Autodesk Inventor part; units mm, degrees
ref_plane "YZ Plane" through (0, 0, 0) normal (1, 0, 0) x (0, 1, 0)
ref_plane "XZ Plane" through (0, 0, 0) normal (0, 1, 0) x (-1, 0, 0)
ref_plane "XY Plane" through (0, 0, 0) normal (0, 0, 1) x (1, 0, 0)
sketch "Sketch1" plane through (0, 0, 0) normal (1, 0, 0) x (0, 1, 0)
  line L0 (0, 0) -> (200, 0)
  line L1 (200, 0) -> (200, -200)
  line L2 (200, -200) -> (0, -200)
  line L3 (0, -200) -> (0, 0)
  dimension "d0" = 200
  dimension "d1" = 200
extrude "Extrusion1" add sketch "Sketch1" along normal blind 6
sketch "Sketch2" plane through (6, 0, 0) normal (1, 0, 0) x (0, 0, -1)
  line L0 (0, 200) -> (0, 0)
  line L1 (0, 0) -> (200, 0)
  line L2 (200, 0) -> (200, 200)
  line L3 (200, 200) -> (0, 200)
  circle A0 centre (50, 130) radius 10
  circle A1 centre (150, 130) radius 10
  circle A2 centre (100, 50) radius 10
  dimension "d4" = 20
  dimension "d5" = 20
  dimension "d6" = 20
  dimension "d7" = 100
  dimension "d8" = 50
  dimension "d9" = 80
  dimension "d10" = 100
  dimension "d11" = 50
  dimension "d12" = 80
extrude "Extrusion2" add sketch "Sketch2" along normal blind 11.1 contours A0 | A1 | A2
sketch "Sketch3" plane through (0, 0, 0) normal (-1, 0, 0) x (0, 0, 1)
  line L0 (0, 0) -> (0, 200)
  line L1 (0, 200) -> (-200, 200)
  line L2 (-200, 200) -> (-200, 0)
  line L3 (-200, 0) -> (0, 0)
  line L4 (-110, 110) -> (-90, 110)
  line L5 (-90, 110) -> (-90, 90)
  line L6 (-90, 90) -> (-110, 90)
  line L7 (-110, 90) -> (-110, 110)
  dimension "d15" = 20
  dimension "d16" = 20
  dimension "d17" = 90
  dimension "d18" = 90
extrude "Extrusion3" add sketch "Sketch3" along normal blind 20 contours L4 L5 L6 L7
sketch "Sketch4" plane through (0, 110, -90) normal (0, 1, 0) x (1, 0, 0)
  line L0 (0, 20) -> (0, 0)
  line L1 (0, 20) -> (-20, 20)
  line L2 (-20, 0) -> (-20, 20)
  line L3 (0, 0) -> (-20, 0)
  line L4 (-20, 0) -> (0, 0)
  line L5 (0, 0) -> (0, 20)
  line L6 (0, 20) -> (-20, 20)
  line L7 (-20, 20) -> (-20, 0)
  point P0 (0, -90)
extrude "Extrusion4" add sketch "Sketch4" along normal blind 200
sketch "Sketch5" plane through (-20, 90, -90) normal (0, 0, 1) x (1, 0, 0)
  line L0 (20, 110) -> (20, 0)
  line L1 (20, 110) -> (20, 220)
  line L2 (0, 220) -> (20, 220)
  line L3 (0, 0) -> (0, 220)
  line L4 (20, 0) -> (0, 0)
  circle A0 centre (10, 180) radius 3.25
  point P0 (20, -90)
  dimension "d23" = 6.5
  dimension "d24" = 40
  dimension "d25" = 10
extrude "Extrusion5" cut sketch "Sketch5" against normal up to next contours A0
properties part number "Arm_Base-Rod-Rev2"
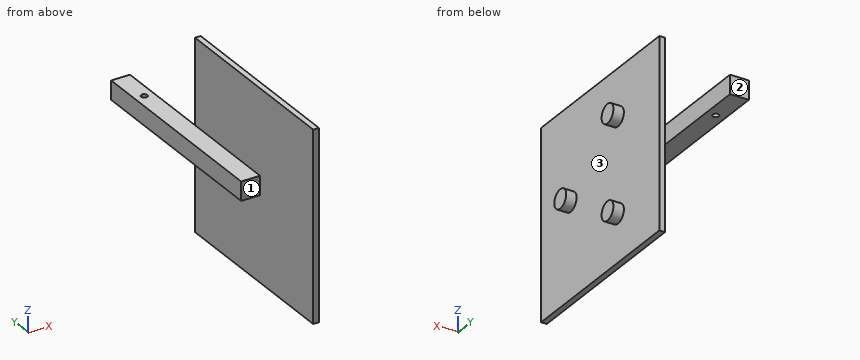
Build history of the part. All positions in model axes, mm. Face numbers are marked on the shaded views. A direction names the side the tool comes from. Give positions to 0.01 mm unless a question says otherwise; leave off trailing zeros. Order: outer loops, then holes, each group sorted by start corner. A loop starts at its lowest first (then second) coordinate and runs counter-clockwise, first axis right, second up. Notation, with made-up numbers: M 4,19.25 L 16,19.25 A10 ccw 16,30.25 Z; hole C 75.5,49.5 d7. An arc over 180 degrees is marked long. Put each result on its own line as item: value.
Item 1: Drop flat-ended pins along their axis: pin 1 Ø5 at (x, y) = (-10, 270) entering from -Z; pin 2 Ø1 at (x, z) = (4.5, -115) entering from +Y; pin 3 Ø10 at (y, z) = (264, -103.5) entering from +X; pin 4 Ø2 at (y, z) = (187.5, -163) entering from +X. Give the stop position or say it passes through.
Results are:
pin 1: through
pin 2: y = 200
pin 3: x = 0
pin 4: x = 6
Item 2: Cut at A-A on x = -10. Write the cut outline in (y, z), then the cut area to 3 significant figures.
Results are:
outline: M 90,-110 L 266.75,-110 L 266.75,-90 L 90,-90 Z; M 273.25,-110 L 310,-110 L 310,-90 L 273.25,-90 Z
area: 4,270 mm2
Item 3: Which spindle directions (+Z, -Z, +X, -X, +Y, -Y) get a long thin tool onto all of the face, cutting with end or side? Do the marked faces 1, 2 and 3. Say none if no direction does.
Results are:
face 1: +Z, -Z, -X, -Y
face 2: +Z, -Z, +X, -X, +Y
face 3: +X
Item 4: Cut at B-B on y = 270. Write the cut outline in (x, z), then the cut area to 3 significant figures.
Results are:
outline: M -20,-110 L -13.25,-110 L -13.25,-90 L -20,-90 Z; M -6.75,-110 L 0,-110 L 0,-90 L -6.75,-90 Z
area: 270 mm2
Item 5: Cut at C-C on z = -100. Write the cut outline in (x, y), then the cut area to 3 significant figures.
Results are:
outline: M -20,90 L 0,90 L 0,0 L 6,0 L 6,40 L 17.1,40 L 17.1,60 L 6,60 L 6,200 L 0,200 L 0,310 L -20,310 Z; hole C -10,270 d6.5
area: 5,790 mm2
Item 6: Wall check: probe 1 along X at (y, z) = (270, -98.75); probe 2 along Y at (x, z) = (-10, -102); probe 3 along X at (y, z) = (193.5, -82). Give the ranges that are in metal, low to high.
Results are:
probe 1: -20 to -13.25, -6.75 to 0
probe 2: 90 to 266.75, 273.25 to 310
probe 3: 0 to 6
Item 7: Cut at D-D on x = 14. Write the cut outline in (y, z), then the cut area to 3 significant figures.
Results are:
outline: C 50,-100 d20; C 130,-150 d20; C 130,-50 d20
area: 942 mm2
